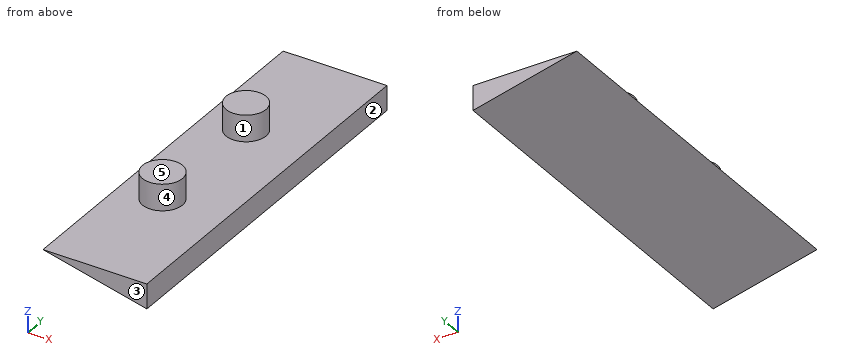
```python
from build123d import *

# Parameters (mm, degrees)
BOSS_EXTRUDE1_DEPTH = 23
SKETCH2_R           = 2.425
BOSS_EXTRUDE2_DEPTH = 3.2


with BuildPart() as part:
    # Sketch1 → Boss-Extrude1 (new, symmetric)
    with BuildSketch(Plane(origin=(0, 0, 0), x_dir=(1, 0, 0), z_dir=(0, 1, 0))):
        Polygon((-6.3, 0), (6.3, 0), (6.3, 3), align=None)
    extrude(amount=BOSS_EXTRUDE1_DEPTH, both=True)

    # Sketch2 → Boss-Extrude2 (add)
    with BuildSketch(Plane.XY):
        with Locations(Location((-1.3, 8, 0), (0, 0, 180))):
            Circle(SKETCH2_R)
        with Locations(Location((-1.3, -8, 0), (0, 0, 180))):
            Circle(SKETCH2_R)
    extrude(amount=BOSS_EXTRUDE2_DEPTH)


solid = part.part
```
CAD build for the part. Positions are in the model's coordinates, mm. Face numbers are marked on the shaded views. A direction names the side the tool comes from. Coordinates: 2 decimals unless noted, no trailing zeros. Order: outer loops, then holes, each group sorted by start corner. A loop starts at its lowest first (then second) coordinate and runs counter-clockwise, first axis right, second up. Notation, with made-up numbers: (35, 57) - (57, 57) arc R21 ccw to (57, 95) - close; hole circle Ø8 at (64.5, 87.5). An arc over 180 degrees is marked (long way). Use a Markdown table: item, result. Add a question column.
(1) Which spindle directions (+Z, -Z, +X, -X, +Y, -Y) get a long thin tool onto all of the face, cutting with end or side? Do the marked faces 1 and 2. Say none if no direction does.
(2) Saw through at D-D (z = 2.75). Give the cut face in (x, y) (3 decimals), then the cut area to 3 significant figures.
(3) Saw through at C-C (x = 0). Give the cut face in (y, z).
(4) Pull direction Y, two halves, no side cores. Call the marked faces 3, 4 and 5: +Y half, -Y half, draft (parallel to the pull), parting line (faces both ways), or undercut.
(5) Flat gauge pins, fed straight in: pin 1 (3 mm diameter, centred on y = -11.5, z = 2, fed in from +X); pin 2 (5 mm diameter, centred on x = -5, y = 15.5, fed in from +Z); pin 3 (6 mm diameter, centred on x = 0.5, y = 18, fed in from -Z). Where does each tip first touch, or does it go through?
(6) Saw through at B-B (z = -2). Give the cut face in (x, y), then the cut area to 3 significant figures.
(7) Drill centre lines: line 1 along Y through (x, z) = (-2.5, 1.5); line 2 along Y through (x, z) = (-2, 2.5); line 3 along Z through (x, y) = (4, -5.5). Where is each one in solid material? Low to high. Write a range as [from, to].
(8) Saw through at A-A (y = -8). Give the cut face in (x, z) (3 decimals), then the cut area to 3 significant figures.
Solved:
| question | item | result |
|---|---|---|
| 1 | face 1 | +Z |
| 1 | face 2 | +Z, -Z, +X, +Y, -Y |
| 2 | outline | circle Ø4.85 at (-1.3, -8); circle Ø4.85 at (-1.3, 8) |
| 2 | area | 36.9 mm² |
| 3 | outline | (-23, -1.5) - (23, -1.5) - (23, 0) - (10.05, 0) - (10.05, 3.2) - (5.95, 3.2) - (5.95, 0) - (-5.95, 0) - (-5.95, 3.2) - (-10.05, 3.2) - (-10.05, 0) - (-23, 0) - close |
| 4 | face 3 | -Y half |
| 4 | face 4 | undercut |
| 4 | face 5 | draft |
| 5 | pin 1 | stops at x = 0.07 |
| 5 | pin 2 | stops at z = 0 |
| 5 | pin 3 | stops at z = -2.33 |
| 6 | outline | (2.1, -23) - (6.3, -23) - (6.3, 23) - (2.1, 23) - close |
| 6 | area | 193 mm² |
| 7 | line 1 | y = [-10.11, -5.89], [5.89, 10.11] |
| 7 | line 2 | y = [-10.32, -5.68], [5.68, 10.32] |
| 7 | line 3 | z = [-2.45, 0] |
| 8 | outline | (-6.3, 0) - (6.3, -3) - (6.3, 0) - (1.125, 0) - (1.125, 3.2) - (-3.725, 3.2) - (-3.725, 0) - close |
| 8 | area | 34.4 mm² |
